Part model, mm, in its own coordinate system. A direction names the side the tool comes from. Give positions to 0.01 mm unless a question says otherwise; leave off trailing zeros. Loops run counter-clockwise (first coordinate to the right, second up) from the corner with the lowest first, then second, coordinate; pieces in that order, holes last. Notation, with made-up numbers: (17.5, 16.25) -> (66.5, 16.25) arc R21 ccw to (66.5, 20.25) -> close; hole circle Ø5 at (11, 22). An arc over 180 degrees is marked (long way). One line per question, with ' | ' between items.
```python
from build123d import *

# Parameters (mm, degrees)
F0_W     = 358.775
F0_H     = 50.8
F1_DEPTH = 12.7
F2_T     = -2.54
F4_DEPTH = 50.801
F5_R     = 2.54
F6_R     = 1.27


with BuildPart() as f1:
    # F0 (on Front) → F1 (new body, symmetric)
    with BuildSketch(Plane.XZ):
        Rectangle(F0_W, F0_H)
    extrude(amount=F1_DEPTH, both=True)

    # F2
    f2_openings = [f1.faces().sort_by_distance(p)[0] for p in [
        (-179.3875, 0, 0),
        (179.3875, 0, 0),
    ]]
    offset(amount=F2_T, openings=f2_openings)

    # F3 (on face) → F4 (cut, through all)
    with BuildSketch(Plane.XY.offset(25.4)):
        Polygon((-179.3875, 12.7), (-179.3875, -12.7), (-109.6015735459, 12.7), align=None)
        Polygon((109.6015735459, 12.7), (179.3875, -12.7), (179.3875, 12.7), align=None)
    extrude(amount=-F4_DEPTH, mode=Mode.SUBTRACT)

    # F5
    f5_edges = [f1.edges().sort_by_distance(p)[0] for p in [
        (0, -12.7, 25.4),
        (0, 12.7, 25.4),
        (0, 12.7, -25.4),
        (0, -12.7, -25.4),
    ]]
    fillet(f5_edges, radius=F5_R)

    # F6
    f6_edges = [f1.edges().sort_by_distance(p)[0] for p in [
        (0, -10.16, -22.86),
        (0, -10.16, 22.86),
        (0, 10.16, 22.86),
        (0, 10.16, -22.86),
    ]]
    fillet(f6_edges, radius=F6_R)


solid = f1.part
```
1) Pin check, flat tips, straight feed: P1, Ø5, axis at x = 138.5, z = -1, coming from the +Y side; P2, Ø12, axis at y = 5, z = -3, coming from the -X side. Stop position of each tip, or through.
Found:
P1: y = -10.16 | P2: x = -116.58
2) Pull direction Y, two halves, no side cores. Call faces 1 (the flat face through (-2, 0, 25.4)), 2 (the flat face through (-3, -12.7, 0)), 3 (the flat face through (-2, 0, 22.86)), 4 (the flat face through (-2, 12.7, 0)): pulls with the +Y half, pulls with the -Y half, needs draft (parallel to the pull), parting line crosses it, or undercut.
Found:
face 1: needs draft | face 2: pulls with the -Y half | face 3: undercut | face 4: pulls with the +Y half
3) Saw through at D-D (x = 150). Give the cut face in (y, z).
Found:
outline: (-12.7, -22.86) arc R2.54 ccw to (-10.16, -25.4) -> (-2, -25.4) -> (-2, -22.86) -> (-8.89, -22.86) arc R1.27 cw to (-10.16, -21.59) -> (-10.16, 21.59) arc R1.27 cw to (-8.89, 22.86) -> (-2, 22.86) -> (-2, 25.4) -> (-10.16, 25.4) arc R2.54 ccw to (-12.7, 22.86) -> close
4) Saw through at C-C (y = 5.75). Give the cut face in (x, z).
Found:
outline: (-128.7, -25.4) -> (128.7, -25.4) -> (128.7, -22.86) -> (-128.7, -22.86) -> close; (-128.7, 22.86) -> (128.7, 22.86) -> (128.7, 25.4) -> (-128.7, 25.4) -> close
5) Saw through at A-A (z = 4). Give the cut face in (x, y), and give its area (3 significant figures).
Found:
outline: (-179.39, -12.7) -> (179.39, -12.7) -> (172.41, -10.16) -> (-172.41, -10.16) -> close; (-116.58, 10.16) -> (116.58, 10.16) -> (109.6, 12.7) -> (-109.6, 12.7) -> close | area: 1,470 mm2
6) Drill centre lines: line 1 (Z direction, x = 1, y = -3); line 2 (Y direction, x = 63, z = -20.5); line 3 (Z direction, x = 50.5, y = 9.25). Where is each one in solid material? Low to high.
Found:
line 1: -25.4 to -22.86, 22.86 to 25.4 | line 2: -12.7 to -10.16, 10.16 to 12.7 | line 3: -25.4 to -22.81, 22.81 to 25.4
7) Saw through at B-B (x = 27). Give the cut face in (y, z), and give its area (3 significant figures).
Found:
outline: (-12.7, -22.86) arc R2.54 ccw to (-10.16, -25.4) -> (10.16, -25.4) arc R2.54 ccw to (12.7, -22.86) -> (12.7, 22.86) arc R2.54 ccw to (10.16, 25.4) -> (-10.16, 25.4) arc R2.54 ccw to (-12.7, 22.86) -> close; hole (-10.16, -21.59) arc R1.27 ccw to (-8.89, -22.86) -> (8.89, -22.86) arc R1.27 ccw to (10.16, -21.59) -> (10.16, 21.59) arc R1.27 ccw to (8.89, 22.86) -> (-8.89, 22.86) arc R1.27 ccw to (-10.16, 21.59) -> close | area: 357 mm2
8) Tool access for faces 5 (the flat face through (-2, 10.16, 0)), 6 (the flat face through (146.916, -0.881, -24.341)): list every direction of +Z, -Z, +X, -X, +Y, -Y with a clear straight run to the whole face (end or side of a thin tool).
Found:
face 5: +X, -X | face 6: +Z, -Z, +X, +Y
